```python
from build123d import *

# Parameters (mm, degrees)
F0_W     = 6
F0_H     = 10
F1_DEPTH = 6


with BuildPart() as f1:
    # F0 (on Top) → F1 (new body)
    with BuildSketch(Plane.XY):
        Polygon((49.193878, -79.867347), (73.193878, -79.867347), (73.193878, -73.867347), (73.193878, -49.867347), (73.193878, -39.867347), (73.193878, 30.132653), (73.193878, 40.132653), (73.193878, 64.132653), (73.193878, 70.132653), (49.193878, 70.132653), (49.193878, 64.132653), (39.193878, 64.132653), (39.193878, 70.132653), (-30.806122, 70.132653), (-30.806122, 64.132653), (-40.806122, 64.132653), (-40.806122, 70.132653), (-64.806122, 70.132653), (-64.806122, 64.132653), (-64.806122, 40.132653), (-64.806122, 30.132653), (-64.806122, -39.867347), (-64.806122, -49.867347), (-64.806122, -73.867347), (-64.806122, -79.867347), (-40.806122, -79.867347), (-40.806122, -73.867347), (-30.806122, -73.867347), (-30.806122, -79.867347), (39.193878, -79.867347), (39.193878, -73.867347), (49.193878, -73.867347), align=None)
        with Locations((-67.806122, 35.132653)):
            Rectangle(F0_W, F0_H)
        with Locations((-67.806122, -44.867347)):
            Rectangle(F0_W, F0_H)
        with Locations((76.193878, -44.867347)):
            Rectangle(F0_W, F0_H)
        with Locations((76.193878, 35.132653)):
            Rectangle(F0_W, F0_H)
    extrude(amount=F1_DEPTH)


solid = f1.part
```
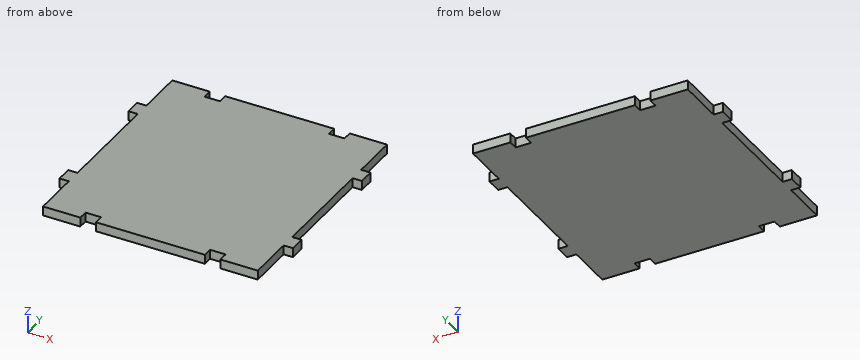
Read the model definition and answer for the solid it produces. Units are mm, in the model's axes. Round coordinates to 2 decimals unless told otherwise and drop trailing zeros. Loops run counter-clockwise (first coordinate to the right, second up) from the corner with the lowest first, then second, coordinate; pieces in that order, holes last. Notation, with made-up numbers: (36.5, -29) -> (57.5, -29) arc R20 cw to (57.5, -15) -> close; hole circle Ø1 at (48.5, 22.5). An arc over 180 degrees is marked (long way). One line per item, written item: value.
1) Consider L1, parallel to X at y = -38, z = 1.3. Determine where the line is inside the solid, lowest interval first. Write a range as [from, to].
Answer list:
L1: x = [-64.81, 73.19]
2) Flat-ended cylindrical pins translate along their axes: P1, Ø3, axis at y = -76, z = 3.5, coming from the +X side; P2, Ø1.8, axis at x = -66.5, z = 2, coming from the -Y side; P3, Ø1.8, axis at y = -66, z = 2.5, coming from the -X side. Find the tip coordinate at first contact, or state that the pin passes through.
Answer list:
P1: stops at x = 73.19
P2: stops at y = -49.87
P3: stops at x = -64.81
3) A cutting plane is placed at A-A (y = -19). Determine the outline of the cut face in (x, z).
Answer list:
outline: (-64.81, 0) -> (73.19, 0) -> (73.19, 6) -> (-64.81, 6) -> close
